```python
from build123d import *

# Parameters (mm, degrees)
SKETCH1_R                 = 3.175
BOSS_EXTRUDE2_DEPTH       = 3.175
F_4_40_TAPPED_HOLE1_D     = 2.2606
F_4_40_TAPPED_HOLE1_DEPTH = 7.62
F_4_40_TAPPED_HOLE1_TIP   = 0.679152758


with BuildPart() as part:
    # Sketch1 → Boss-Extrude2 (new body, symmetric)
    with BuildSketch(Plane(origin=(0, 0, 0), x_dir=(0, 0, -1), z_dir=(1, 0, 0))):
        with BuildLine():
            Line((25.4, -50.8), (25.4, -38.1))
            Line((25.4, -38.1), (22.225, -38.1))
            Line((22.225, -38.1), (22.225, -41.275))
            Line((22.225, -41.275), (19.05, -41.275))
            Line((19.05, -41.275), (19.05, -38.1))
            Line((19.05, -38.1), (0, -38.1))
            ThreePointArc((0, -38.1), (-38.1, 0), (0, 38.1))
            ThreePointArc((0, 38.1), (67.501425911, 12.737343898), (101.6, -50.8))
            Line((101.6, -50.8), (241.3, -50.8))
            Line((241.3, -50.8), (241.3, 60.325))
            Line((241.3, 60.325), (228.6, 60.325))
            Line((228.6, 60.325), (228.6, 57.15))
            Line((228.6, 57.15), (215.9, 57.15))
            Line((215.9, 57.15), (215.9, 60.325))
            Line((215.9, 60.325), (184.15, 60.325))
            Line((184.15, 60.325), (184.15, 57.15))
            Line((184.15, 57.15), (171.45, 57.15))
            Line((171.45, 57.15), (171.45, 60.325))
            Line((171.45, 60.325), (0, 60.325))
            add(Edge.make_bspline(
                [(-27.840906439, 52.6855483), (-15.97034645, 60.327815279), (0, 60.325)],
                knots=[0.821555454, 0.821555454, 0.821555454, 1, 1, 1], degree=2))
            add(Edge.make_bspline(
                [(-58.625125689, 0), (-58.995342849, 19.785116254), (-54.931758321, 37.043947765), (-27.840906439, 52.6855483)],
                knots=[0.494452285, 0.494452285, 0.494452285, 0.494452285, 0.821555454, 0.821555454, 0.821555454, 0.821555454], degree=3))
            add(Edge.make_bspline(
                [(-41.752199567, -38.1), (-52.707301474, -27.360886787), (-58.323372846, -16.126251656), (-58.625125689, 0)],
                knots=[0.219145, 0.219145, 0.219145, 0.219145, 0.494452285, 0.494452285, 0.494452285, 0.494452285], degree=3))
            add(Edge.make_bspline(
                [(0, -50.8), (-28.671783901, -50.922524692), (-41.752199567, -38.1)],
                knots=[0, 0, 0, 0.219145, 0.219145, 0.219145], degree=2))
            Line((0, -50.8), (25.4, -50.8))
        make_face()
        with Locations((231.775, 4.7625)):
            Circle(SKETCH1_R, mode=Mode.SUBTRACT)
    extrude(amount=BOSS_EXTRUDE2_DEPTH, both=True)

    # #4-40 Tapped Hole1
    with Locations(Plane(origin=(0, 57.15, 0), x_dir=(1, 0, 0), z_dir=(0, 1, 0))):
        with Locations((0, 177.8), (0, 222.25)):
            Hole(F_4_40_TAPPED_HOLE1_D / 2, depth=F_4_40_TAPPED_HOLE1_DEPTH)
            with Locations((0, 0, -(F_4_40_TAPPED_HOLE1_DEPTH + F_4_40_TAPPED_HOLE1_TIP / 2))):  # 118° drill point
                Cone(0, F_4_40_TAPPED_HOLE1_D / 2, F_4_40_TAPPED_HOLE1_TIP, mode=Mode.SUBTRACT)


solid = part.part
```
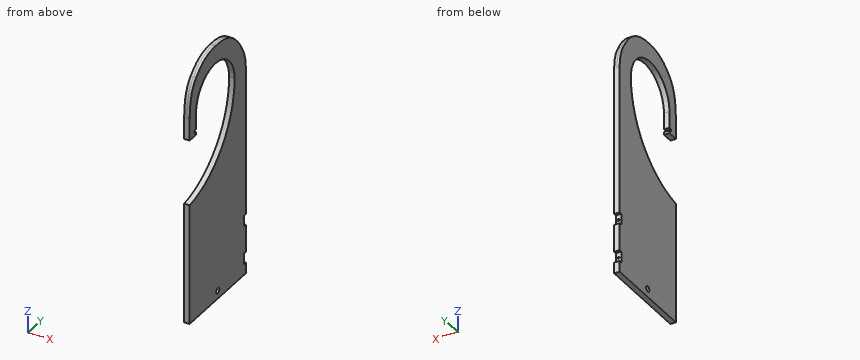
For this review, take the finished solid that the model builds, in its own axes (mm). Give positions to 0.01 mm unless a question says otherwise; leave off trailing zeros. Order: outer loops, then holes, each group sorted by start corner. A loop starts at its lowest first (then second) coordinate and runs counter-clockwise, first axis right, second up.
1) Take a section at B-B (z = -46.5). Give the boundary of the cut face in (x, y) (3 decimals).
2) Take a section at A-A (z = -78). Give the boundary of the cut face in (x, y) (3 decimals).
3) Insertion check: pin 1 (2 mm diameter, centred on x = 1.5, z = -50, fed in from -Y); pin 2 (6 mm diameter, centred on y = -11.5, z = -86, fed in from -X) (3 decimals); pin 3 (2 mm diameter, centred on x = -2, y = 41, fed in from +Z); pin 4 (1.8 mm diameter, centred on x = 0, z = -222.25, fed in from +Y). Each pin has a flat end and moves straight along its axis. Give the tip position at first contact, or say it passes through.
4) Wall thickness on line 1 (X direction, y = 54.5, z = -177.8) (3 decimals); line 2 (Z direction, x = -0.75, y = 53); line 3 (Z direction, x = 0, y = 53): over which ranges is each line inside the solid? List them lowest first.
Derived:
1. outline: (-3.175, 26.946) - (3.175, 26.946) - (3.175, 60.325) - (-3.175, 60.325) - close
2. outline: (-3.175, 2.104) - (3.175, 2.104) - (3.175, 60.325) - (-3.175, 60.325) - close
3. pin 1: stops at y = 24.51
3. pin 2: stops at x = -3.175
3. pin 3: stops at z = 44.77
3. pin 4: stops at y = 49.39
4. line 1: x = -3.175 to -1.13, 1.13 to 3.175
4. line 2: z = -241.3 to -223.1, -221.4 to -178.65, -176.95 to 27.35
4. line 3: z = -241.3 to -223.38, -221.12 to -178.93, -176.67 to 27.35
